```python
from build123d import *

# Parameters (mm, degrees)
F3_R = 5.08


# Not quite as in the source:
# - a variable given as a bare number and used for a length is read in inches; the dataset says mm whatever the document's units were


with BuildPart() as f2:
    # F1 (on Front) → F2 (revolve)
    with BuildSketch(Plane.XZ):
        Polygon((-25.4, 46.355), (0, 31.75), (50.8, 32.385), (50.8, 36.195), (0, 36.195), (-25.4, 50.38725), (-28.575, 53.56225), (-31.75, 50.38725), (-76.2, 50.165), (-76.2, 46.355), align=None)
    revolve(axis=Axis((-24.3991323134, 0, 0), (-1, 0, 0)))

    # F3
    f3_edges = [f2.edges().sort_by_distance(p)[0] for p in [
        (-25.4, 0, -46.355),
        (0, 0, -31.75),
        (0, 0, -36.195),
        (-31.75, 0, -50.38725),
        (-25.4, 0, -50.38725),
    ]]
    fillet(f3_edges, radius=F3_R)


solid = f2.part
```
CAD build for the part. Positions are in the model's coordinates, mm. A direction names the side the tool comes from. Give positions to 0.01 mm unless a question says otherwise; leave off trailing zeros. Loops run counter-clockwise (first coordinate to the right, second up) from the corner with the lowest first, then second, coordinate; pieces in that order, holes last. Notation, with made-up numbers: M 72.25,35.5 L 80.25,35.5 A35 cw 80.25,73.5 Z; hole C 58,84.5 d10. An arc over 180 degrees is marked long. Use one line per item in the form item = value.
Item 1: Drill centre lines: probe 1 along Z at (x, y) = (-38, 0) (3 decimals); probe 2 along Y at (x, z) = (-65.5, 1); probe 3 along Z at (x, y) = (-54.5, 0) (1 decimal). Where is each one in solid material? Low to high. Write a range as from..to.
Determined:
probe_1 = -50.356..-46.355, 46.355..50.356
probe_2 = -50.21..-46.34, 46.34..50.21
probe_3 = -50.3..-46.4, 46.4..50.3
Item 2: Flat gauge pins, fed straight in: pin 1 (2 mm diameter, centred on x = -28.5, z = 15, fed in from +Y); pin 2 (1.5 mm diameter, centred on y = -31, z = 23, fed in from +X); pin 3 (8 mm diameter, centred on x = 24.5, y = 42.5, fed in from +Z); pin 4 (4 mm diameter, centred on y = 27, z = -32.5, fed in from -X). Where does each tip first touch, or does it go through?
Determined:
pin_1 = 51.7
pin_2 = -2.96
pin_3 = through
pin_4 = -21.74
Item 3: Which spindle directions (+Z, -Z, +X, -X, +Y, -Y) get a long thin tool onto all of the face, cutting with end or side? Do faces 1 (the face through (-76.2, -14.6, 44.4)), 2 (the face through (-55.32, -30.59, -39.89)), 3 (the face through (26.441, -12.287, 29.634)). Say none if no direction does.
Determined:
face_1 = +Z, -Z, -X, +Y, -Y
face_2 = -X
face_3 = +X
Item 4: Two-plate mould, pull along Z, no slides. Class faces 4 (the face through (50.8, -19, 27)), 5 (the face through (25.715, -22.024, -28.723)), 6 (the face through (-51.1, -17.8, 42.8)): pulls with the +Z half, pulls with the -Z half, needs draft (parallel to the pull), parting line crosses it, or undercut.
Determined:
face_4 = needs draft
face_5 = parting line crosses it
face_6 = undercut
Item 5: Slice it at B-B (x = -52). List the corners of the cut face in (y, z) (3 decimals).
Determined:
outline = C 0,0 d100.572; hole C 0,0 d92.71
Item 6: Slice it at A-A (x = -22). List the corners of the cut face in (y, z) (1 decimal), plus the area to 3 significant figures.
Determined:
outline = C 0,0 d97; hole C 0,0 d88.8
area = 1,190 mm2
